Could you check a few things on this model? Use its own coordinates, in mm. A direction names the side the tool comes from. Round coordinates to 2 decimals unless told otherwise and drop trailing zeros. Loops run counter-clockwise (first coordinate to the right, second up) from the corner with the lowest first, then second, coordinate; pieces in that order, holes last. Notation, with made-up numbers: (81, -35.5) -> (122, -35.5) arc R25 cw to (122, 0.5) -> close; hole circle Ø4 at (54, 75). An arc over 180 degrees is marked (long way). One line per item, written item: value.
```python
from build123d import *

# Parameters (mm, degrees)
SKETCH029_R     = 1.6
PAD013_DEPTH    = 6
POCKET001_DEPTH = 6.001
POCKET002_DEPTH = 6.001
PAD014_DEPTH    = 1.5
PAD015_DEPTH    = 20
SKETCH034_W     = 0.2
SKETCH034_H     = 14
POCKET003_DEPTH = 1.5
SKETCH035_W     = 0.2
SKETCH035_H     = 14
POCKET004_DEPTH = 1.5
SKETCH036_R     = 1.6
PAD016_DEPTH    = 17
POCKET005_DEPTH = 11.8810475508
POCKET006_DEPTH = 6.251
FILLET001_R     = 1


with BuildPart() as part:
    # Sketch029 (on Face1 of Binder) → Pad013 (new body)
    with BuildSketch(Plane.XY.offset(3)):
        with BuildLine():
            Line((-66.15, -41.34), (-56.1, -41.34))
            Line((-56.1, -41.34), (-56.1, -37.84))
            ThreePointArc((-52.6, -34.34), (-55.0748725626, -35.3651274374), (-56.1, -37.84))
            Line((-52.6, -34.34), (-49.1, -34.34))
            Line((-49.1, -34.34), (-49.1, 17.6675))
            Line((-49.1, 17.6675), (-37.05, 17.6675))
            Line((-37.05, 17.6675), (-37.05, 20.525))
            ThreePointArc((-30.05, 20.525), (-33.55, 24.025), (-37.05, 20.525))
            Line((-30.05, 20.525), (-11.725, 20.525))
            Line((-11.725, 20.525), (-11.725, 30.775))
            Line((-11.725, 30.775), (11.725, 30.775))
            Line((11.725, 30.775), (11.725, 20.4910582095))
            Line((11.725, 20.4910582095), (33.4250449924, 18.9736432442))
            Line((33.4250449924, 18.9736432442), (32.8973962111, 11.4279141223))
            Line((32.8973962111, 11.4279141223), (36.3697437262, 11.1851039306))
            ThreePointArc((39.5724232036, 7.0858611329), (38.8836355297, 9.8484463434), (36.3697437262, 11.1851039306))
            Line((39.5724232036, 7.0858611329), (38.9679840019, 3.657916077))
            Line((38.9679840019, 3.657916077), (55.7764699529, 0.694126499))
            Line((55.7764699529, 0.694126499), (54.2483659895, -7.9721817275))
            Line((54.2483659895, -7.9721817275), (73.7229393053, -11.4060744409))
            Line((73.7229393053, -11.4060744409), (66.3428917544, -53.2604039439))
            Line((66.3428917544, -53.2604039439), (53.7619727097, -51.0420484742))
            Line((53.5362300787, -52.3222985531), (53.7619727097, -51.0420484742))
            ThreePointArc((49.4816343214, -55.1613570668), (52.0969209571, -54.5815627814), (53.5362300787, -52.3222985531))
            Line((46.0348071858, -54.553588445), (49.4816343214, -55.1613570668))
            Line((46.0348071858, -54.553588445), (45.3402144751, -58.492819457))
            Line((45.3402144751, -58.492819457), (23.6744439088, -54.6725595483))
            Line((23.6744439088, -54.6725595483), (26.1271109464, -40.7627935689))
            Line((26.1271109464, -40.7627935689), (7.2862718147, -39.4453137541))
            Line((7.2862718147, -39.4453137541), (7.9432561527, -30.05))
            Line((7.9432561527, -30.05), (-0.05, -30.05))
            Line((-0.05, -30.05), (-0.05, -33.55))
            ThreePointArc((-3.55, -37.05), (-1.0751246396, -36.0248753604), (-0.05, -33.55))
            Line((-3.55, -37.05), (-7.05, -37.05))
            Line((-7.05, -37.05), (-7.05, -62.34))
            Line((-9.525, -62.34), (-7.05, -62.34))
            Line((-9.525, -21.9075), (-9.525, -62.34))
            Line((9.9912370186, -21.9075), (-9.525, -21.9075))
            Line((8.8605695876, -38.0767975787), (9.9912370186, -21.9075))
            Line((27.864164745, -39.4056584035), (8.8605695876, -38.0767975787))
            Line((25.3831664066, -53.4760991747), (27.864164745, -39.4056584035))
            Line((44.1437541015, -56.7840969593), (25.3831664066, -53.4760991747))
            Line((45.7977529938, -47.4038031118), (44.1437541015, -56.7840969593))
            Line((64.5583406887, -50.7118008964), (45.7977529938, -47.4038031118))
            Line((71.1743362578, -13.1906255066), (64.5583406887, -50.7118008964))
            Line((52.4137485629, -9.8826277221), (71.1743362578, -13.1906255066))
            Line((54.0677474552, -0.5023338746), (52.4137485629, -9.8826277221))
            Line((30.870571009, 3.5879542091), (54.0677474552, -0.5023338746))
            Line((31.8507472195, 17.6051270688), (30.870571009, 3.5879542091))
            Line((9.525, 19.1662953961), (31.8507472195, 17.6051270688))
            Line((9.525, 28.575), (9.525, 19.1662953961))
            Line((-9.525, 28.575), (9.525, 28.575))
            Line((-9.525, 19.05), (-9.525, 28.575))
            Line((-28.575, 19.05), (-9.525, 19.05))
            Line((-28.575, 16.1925), (-28.575, 19.05))
            Line((-47.625, 16.1925), (-28.575, 16.1925))
            Line((-47.625, -43.815), (-47.625, 16.1925))
            Line((-66.15, -43.815), (-47.625, -43.815))
            Line((-66.15, -41.34), (-66.15, -43.815))
        make_face()
        with Locations((-33.55, 20.525)):
            Circle(SKETCH029_R, mode=Mode.SUBTRACT)
        with Locations((-52.599996, -37.840004)):
            Circle(SKETCH029_R, mode=Mode.SUBTRACT)
        with Locations((-3.5499944477, -33.5500055523)):
            Circle(SKETCH029_R, mode=Mode.SUBTRACT)
        with Locations((50.0894046049, -51.7145323045)):
            Circle(SKETCH029_R, mode=Mode.SUBTRACT)
        with Locations((36.1256015808, 7.6936340617)):
            Circle(SKETCH029_R, mode=Mode.SUBTRACT)
    extrude(amount=PAD013_DEPTH)

    # Sketch030 (on Vertex106 of Pad013) → Pocket001 (cut, through all)
    with BuildSketch(Plane(origin=(9.525, 28.575, 9), x_dir=(1, 0, 0), z_dir=(0, 0, 1))):
        Polygon((0, 0), (0, -19.05), (0.2, -19.05), (0.2, 0.2), (-19.25, 0.2), (-19.25, -19.05), (-19.05, -19.05), (-19.05, 0), align=None)
    extrude(amount=-POCKET001_DEPTH, mode=Mode.SUBTRACT)

    # Sketch031 (on Vertex111 of Pocket001) → Pocket002 (cut, through all)
    with BuildSketch(Plane(origin=(64.5583406887, -50.7118008964, 9), x_dir=(1, 0, 0), z_dir=(0, 0, 1))):
        Polygon((6.6159955691, 37.5211753898), (0, 0), (-18.7605876949, 3.3079977846), (-18.7953173304, 3.111036234), (0.1622319151, -0.2316911861), (6.8476867552, 37.6834073048), (-12.1098624902, 41.0261347249), (-12.1445921258, 40.8291731743), align=None)
    extrude(amount=-POCKET002_DEPTH, mode=Mode.SUBTRACT)

    # Sketch032 (on Face5 of Pocket002) → Pad014 (join)
    with BuildSketch(Plane(origin=(0, 0, 9), x_dir=(-1, 0, 0), z_dir=(0, 0, -1))):
        Polygon((11.725, 26.025), (11.725, 19.05), (28.575, 19.05), (28.575, 16.1925), (47.625, 16.1925), (47.625, -43.815), (66.15, -43.815), (66.15, 26.025), align=None)
        Polygon((-11.725, 26.025), (-63.3428917544, 26.025), (-63.3428917544, -11.6066452204), (-52.4484781984, -9.6856661715), (-54.0677474552, -0.5023338746), (-30.870571009, 3.5879542091), (-31.8507472195, 17.6051270688), (-11.725, 19.0124564098), align=None)
        Polygon((9.525, -62.34), (9.525, -21.9075), (-9.9912370186, -21.9075), (-8.8605695876, -38.0767975787), (-27.864164745, -39.4056584035), (-25.3831664066, -53.4760991747), (-44.1437541015, -56.7840969593), (-45.7630233582, -47.6007646624), (-63.3428917544, -50.700569778), (-63.3428917544, -62.34), align=None)
    extrude(amount=PAD014_DEPTH)

    # Sketch033 (on Face78 of Pad014) → Pad015 (join)
    with BuildSketch(Plane(origin=(0, 0, 9), x_dir=(-1, 0, 0), z_dir=(0, 0, -1))):
        Polygon((66.15, -41.34), (66.15, 26.025), (11.725, 26.025), (11.725, 30.775), (-11.725, 30.775), (-11.725, 26.025), (-63.3428917544, 26.025), (-63.3428917544, -9.5757919966), (-73.7229393053, -11.4060744409), (-66.3428917544, -53.2604039439), (-63.3428917544, -52.7314230018), (-63.3428917544, -62.34), (7.05, -62.34), (7.05, -60.84), (-61.8428917544, -60.84), (-61.8428917544, -50.4360793069), (-64.7205726037, -50.9434920825), (-71.4060274439, -13.0283935916), (-61.8428917544, -11.3421547493), (-61.8428917544, 24.525), (-9.725, 24.525), (-9.725, 28.775), (9.725, 28.775), (9.725, 24.525), (64.65, 24.525), (64.65, -41.34), align=None)
    extrude(amount=PAD015_DEPTH)

    # Sketch034 (on Vertex1 of Pad015) → Pocket003 (cut)
    with BuildSketch(Plane(origin=(-66.15, -41.34, 3), x_dir=(0, -1, 0), z_dir=(-1, 0, 0))):
        with Locations((-0.1, -7)):
            Rectangle(SKETCH034_W, SKETCH034_H)
    extrude(amount=-POCKET003_DEPTH, mode=Mode.SUBTRACT)

    # Sketch035 → Pocket004 (cut)
    with BuildSketch(Plane(origin=(-7.05, -62.34, 3), x_dir=(1, 0, 0), z_dir=(0, -1, 0))):
        with Locations((0.1, -7)):
            Rectangle(SKETCH035_W, SKETCH035_H)
    extrude(amount=-POCKET004_DEPTH, mode=Mode.SUBTRACT)

    # Sketch036 (on Face27 of Pocket004) → Pad016 (join)
    with BuildSketch(Plane.XY.offset(9)):
        with BuildLine():
            Line((-64.65, 24.525), (-57.65, 24.525))
            Line((-57.65, 24.525), (-57.65, 21.025))
            ThreePointArc((-61.15, 17.525), (-58.6751262658, 18.5501262658), (-57.65, 21.025))
            Line((-64.65, 17.525), (-61.15, 17.525))
            Line((-64.65, 24.525), (-64.65, 17.525))
        make_face()
        with Locations((-61.15, 21.025)):
            Circle(SKETCH036_R, mode=Mode.SUBTRACT)
        with BuildLine():
            Line((-64.65, -34.14), (-64.65, -41.14))
            Line((-64.65, -41.14), (-61.15, -41.14))
            ThreePointArc((-61.15, -41.14), (-57.65, -37.64), (-61.15, -34.14))
            Line((-64.65, -34.14), (-61.15, -34.14))
        make_face()
        with Locations((-61.15, -37.64)):
            Circle(SKETCH036_R, mode=Mode.SUBTRACT)
        with BuildLine():
            Line((61.8428917544, -53.84), (61.8428917544, -60.84))
            Line((61.8428917544, -60.84), (54.8428917544, -60.84))
            Line((54.8428917544, -60.84), (54.8428917544, -57.34))
            ThreePointArc((58.3428917544, -53.84), (55.8680180203, -54.8651262658), (54.8428917544, -57.34))
            Line((61.8428917544, -53.84), (58.3428917544, -53.84))
        make_face()
        with Locations((58.3428917544, -57.34)):
            Circle(SKETCH036_R, mode=Mode.SUBTRACT)
        with BuildLine():
            Line((61.8428917544, 24.525), (61.8428917544, 17.525))
            Line((61.8428917544, 17.525), (58.3428917544, 17.525))
            ThreePointArc((54.8428917544, 21.025), (55.8680180203, 18.5501262658), (58.3428917544, 17.525))
            Line((54.8428917544, 24.525), (54.8428917544, 21.025))
            Line((54.8428917544, 24.525), (61.8428917544, 24.525))
        make_face()
        with Locations((58.3428917544, 21.025)):
            Circle(SKETCH036_R, mode=Mode.SUBTRACT)
    extrude(amount=-PAD016_DEPTH)

    # Sketch037 (on Vertex85 of Pad016) → Pocket005 (cut, through all)
    with BuildSketch(Plane(origin=(61.8428917544, 16.525, -11), x_dir=(0, 1, 0), z_dir=(1, 0, 0))):
        with BuildLine():
            Line((0, 0), (0, 3))
            Line((-5.5, 3), (0, 3))
            Line((-5.5, 3.6), (-5.5, 3))
            ThreePointArc((-5.5, 3.6), (-5.9100505063, 4.5899494937), (-6.9, 5))
            Line((-13.4, 5), (-6.9, 5))
            ThreePointArc((-13.4, 5), (-14.3899494937, 4.5899494937), (-14.8, 3.6))
            Line((-14.8, 3), (-14.8, 3.6))
            Line((-20.3, 3), (-14.8, 3))
            Line((-20.3, 3), (-20.3, 0))
            Line((-20.3, 0), (0, 0))
        make_face()
    extrude(amount=POCKET005_DEPTH, mode=Mode.SUBTRACT)

    # Sketch038 (on Vertex75 of Pocket005) → Pocket006 (cut, through all)
    with BuildSketch(Plane(origin=(48.8428917544, 24.525, -11), x_dir=(1, 0, 0), z_dir=(0, -1, 0))):
        with BuildLine():
            ThreePointArc((-3.6, 7), (-7, 10.4), (-10.4, 7))
            Line((-10.4, 7), (-10.4, 0))
            Line((-10.4, 0), (-3.6, 0))
            Line((-3.6, 0), (-3.6, 7))
        make_face()
    extrude(amount=-POCKET006_DEPTH, mode=Mode.SUBTRACT)

    # Fillet001
    fillet001_edges = [part.edges().sort_by_distance(p)[0] for p in [
        (-9.525, -62.34, 6),
        (-66.15, -43.815, 6),
        (63.342892, -62.34, -1),
        (66.342892, -53.260404, -1),
        (73.722939, -11.406074, -1),
        (63.342892, 26.025, -1),
        (-66.15, 26.025, -1),
        (-11.725, 30.775, -1),
        (11.725, 30.775, -1),
    ]]
    fillet(fillet001_edges, radius=FILLET001_R)


solid = part.part
```
(1) We'd pull the mould along X, two halves only. Please class faces 4 (the face through (-52, -3, 7.5)), 5 (the face through (11.725, 23, 5)), 6 (the face through (0, 30.775, -1)): +X half, -X half, draft (parallel to the pull), parting line (faces both ways), or undercut.
Results below:
face 4: undercut
face 5: undercut
face 6: draft
(2) For pin 1 Ø10 at (x, y) = (-12, 14.5) entering from -Z; pin 2 Ø8 at (x, z) = (47.5, -6) entering from +Y (3 decimals); pin 3 Ø10 at (y, z) = (-40.5, -7.5) entering from +X, each with a flat end and sliding along its axis, tell me the tip position at first contact or that it passes through.
Results below:
pin 1: stops at z = 3
pin 2: stops at y = 26.025
pin 3: stops at x = 69.47
(3) Please list where these lines run through material, in increasing order: L1, parallel to Y at x = -61.15, z = -3 (3 decimals); L2, parallel to Y at x = 13, z = -5.75 (3 decimals); L3, parallel to X at y = -7, z = 1.5.
Results below:
L1: y = -41.14 to -39.24, -36.04 to -34.14, 17.525 to 19.425, 22.625 to 26.025
L2: y = -62.34 to -60.84, 24.525 to 26.025
L3: x = -66.15 to -64.65, 61.84 to 63.34
(4) Imagine slicing it at C-C on y = -2. Write out the boundary of the cut face in (x, z) (3 decimals), then the cut area to 3 significant figures.
Results below:
outline: (-66.15, -11) -> (-64.65, -11) -> (-64.65, 7.5) -> (-49.1, 7.5) -> (-49.1, 3) -> (-47.625, 3) -> (-47.625, 9) -> (-66.15, 9) -> close; (53.804, 3) -> (55.301, 3) -> (55.301, 7.5) -> (61.843, 7.5) -> (61.843, -8) -> (63.343, -8) -> (63.343, 9) -> (53.804, 9) -> close
area: 106 mm²
(5) Imagine slicing it at A-A on y = -23.5. Write out the boundary of the cut face in (x, z) (3 decimals), then the cut area to 3 significant figures.
Results below:
outline: (-66.15, -11) -> (-64.65, -11) -> (-64.65, 7.5) -> (-49.1, 7.5) -> (-49.1, 3) -> (-47.625, 3) -> (-47.625, 9) -> (-66.15, 9) -> close; (-9.525, 3) -> (9.88, 3) -> (9.88, 9) -> (-9.525, 9) -> close; (69.56, -11) -> (71.59, -11) -> (71.59, 9) -> (69.56, 9) -> close
area: 219 mm²
(6) On a 3-axis mill with a long thin cutter (end or side, diameter ignored), from which of +Z, -Z, +X, -X, +Y, -Y can I reach the whole of each face in a straight line? I mean faces 1 (the face through (18.5, -38.75, 5.96)), 2 (the face through (27, -60.84, -2)), 3 (the face through (-9.725, 25, 1)). Say none if no direction works.
Results below:
face 1: +Z, -Z
face 2: -Z
face 3: +Z, -Z, -Y
(7) Imagine slicing it at B-B on x = -41. Write out the boundary of the cut face in (y, z) (1 decimal).
Results below:
outline: (16.2, 3) -> (17.7, 3) -> (17.7, 7.5) -> (24.5, 7.5) -> (24.5, -11) -> (26, -11) -> (26, 9) -> (16.2, 9) -> close
